```python
from build123d import *

# Parameters (mm, degrees)
BOSS_EXTRUDE1_DEPTH = 22
SKETCH2_R           = 3
BOSS_EXTRUDE2_DEPTH = 14
SKETCH5_R           = 3.63
BOSS_EXTRUDE3_DEPTH = 2
SKETCH7_R           = 1.5
CUT_EXTRUDE1_DEPTH  = 3.5
SKETCH8_R           = 12
BOSS_EXTRUDE4_DEPTH = 31
SKETCH9_R           = 1.5
BOSS_EXTRUDE5_DEPTH = 7
SKETCH10_R          = 4
BOSS_EXTRUDE6_DEPTH = 2
SKETCH11_R          = 1.5
CUT_EXTRUDE2_DEPTH  = 3.5


with BuildPart() as part:
    # Sketch1 → Boss-Extrude1 (new body)
    with BuildSketch(Plane.XY):
        with BuildLine():
            Line((-20.5, -16), (20.5, -16))
            ThreePointArc((20.5, -16), (22.267766953, -15.267766953), (23, -13.5))
            Line((23, -13.5), (23, 13.5))
            ThreePointArc((23, 13.5), (22.267766953, 15.267766953), (20.5, 16))
            Line((20.5, 16), (-20.5, 16))
            ThreePointArc((-20.5, 16), (-22.267766953, 15.267766953), (-23, 13.5))
            Line((-23, 13.5), (-23, -13.5))
            ThreePointArc((-23, -13.5), (-22.267766953, -15.267766953), (-20.5, -16))
        make_face()
    extrude(amount=BOSS_EXTRUDE1_DEPTH)

    # Sketch2 → Boss-Extrude2 (add)
    with BuildSketch(Plane.XY.offset(22)):
        with Locations((-8.2, 0)):
            Circle(SKETCH2_R)
    extrude(amount=BOSS_EXTRUDE2_DEPTH)

    # Sketch5 → Boss-Extrude3 (add)
    with BuildSketch(Plane.XY.offset(22)):
        with Locations((-17.2, 9.11)):
            Circle(SKETCH5_R)
        with Locations((-17.2, -9.09)):
            Circle(SKETCH5_R)
        with Locations((15.8, 9.11)):
            Circle(SKETCH5_R)
        with Locations((15.8, -9.09)):
            Circle(SKETCH5_R)
    extrude(amount=BOSS_EXTRUDE3_DEPTH)

    # Sketch7 → Cut-Extrude1 (cut)
    with BuildSketch(Plane.XY.offset(24)):
        with Locations((-17.2, 9.11)):
            Circle(SKETCH7_R)
        with Locations((-17.2, -9.09)):
            Circle(SKETCH7_R)
        with Locations((15.7, 9.11)):
            Circle(SKETCH7_R)
        with Locations((15.7, -9.09)):
            Circle(SKETCH7_R)
    extrude(amount=-CUT_EXTRUDE1_DEPTH, mode=Mode.SUBTRACT)

    # Sketch8 → Boss-Extrude4 (add)
    with BuildSketch(Plane(origin=(23, 0, 0), x_dir=(0, 0, -1), z_dir=(1, 0, 0))):
        with Locations(Location((-10, 0, 0), (0, 0, 180))):
            Circle(SKETCH8_R)
    extrude(amount=BOSS_EXTRUDE4_DEPTH)

    # Sketch9 → Boss-Extrude5 (add)
    with BuildSketch(Plane(origin=(54, 0, 0), x_dir=(0, 0, -1), z_dir=(1, 0, 0))):
        with Locations((-10, 0)):
            Circle(SKETCH9_R)
    extrude(amount=BOSS_EXTRUDE5_DEPTH)

    # Sketch10 → Boss-Extrude6 (add)
    with BuildSketch(Plane(origin=(57, 0, 0), x_dir=(0, 0, -1), z_dir=(1, 0, 0))):
        with Locations((-10, 0)):
            Circle(SKETCH10_R)
    extrude(amount=BOSS_EXTRUDE6_DEPTH)

    # Sketch11 → Cut-Extrude2 (cut)
    with BuildSketch(Plane.XY.offset(36)):
        with Locations((-8.2, 0)):
            Circle(SKETCH11_R)
    extrude(amount=-CUT_EXTRUDE2_DEPTH, mode=Mode.SUBTRACT)


solid = part.part
```
Geometry check sheet. Reference: the model listing, model coordinates, mm. A direction names the side the tool comes from. Round coordinates to 2 decimals unless told otherwise and drop trailing zeros. Loops run counter-clockwise (first coordinate to the right, second up) from the corner with the lowest first, then second, coordinate; pieces in that order, holes last. Notation, with made-up numbers: (-21, 10.25) -> (36, 10.25) arc R18 cw to (36, 45.25) -> close; hole circle Ø6 at (40, 60.5). An arc over 180 degrees is marked (long way). Use a Markdown table: item, result.
(1) Set-up check for faces 1 (the flat face through (57, -2, 10)), 2 (the cylindrical face through (38.28, -0.53, -1.99)), 3 (the cylindrical face through (-22.287, -15.248, 10.846)), 4 (the cylindrical face through (-15.52, -12.31, 22.99)), 5 (the flat face through (0, -16, 11)): record each of +Z, -Z, +X, -X, +Y, -Y from which the full face is reachable in a straight line by a thin tool's end or side.
Calculated:
| item | result |
|---|---|
| face 1 | none |
| face 2 | +X |
| face 3 | +Z, -Z, -X, -Y |
| face 4 | +Z |
| face 5 | +Z, -Z, +X, -X, -Y |
(2) Go/stop test with flat-tipped pins: P1, Ø3.5, axis at x = -17.5, y = -9, coming from the +Z side; P2, Ø10, axis at x = 15, y = 5.5, coming from the -Z side; P3, Ø6, axis at x = 49, z = 20, coming from the +Y side. Record where each tip stops, or that it passes through.
Calculated:
| item | result |
|---|---|
| P1 | z = 24 |
| P2 | z = 0 |
| P3 | y = 9.75 |
(3) Sectioned sample at A-A (x = -17.2). Enter the section's corners in (y, z), then the cut area to 3 significant figures.
Calculated:
| item | result |
|---|---|
| outline | (-16, 0) -> (16, 0) -> (16, 22) -> (12.74, 22) -> (12.74, 24) -> (10.61, 24) -> (10.61, 20.5) -> (7.61, 20.5) -> (7.61, 24) -> (5.48, 24) -> (5.48, 22) -> (-5.46, 22) -> (-5.46, 24) -> (-7.59, 24) -> (-7.59, 20.5) -> (-10.59, 20.5) -> (-10.59, 24) -> (-12.72, 24) -> (-12.72, 22) -> (-16, 22) -> close |
| area | 712 mm² |
(4) Mould release check, pull along Y, two halves, no side actions. Record for faces 6 (the flat face through (54, 2, 10)), 7 (the flat face through (16, -9, 20.5)), 8 (the cylindrical face through (22.248, -15.287, 10.846)): released by +Y, released by -Y, zero draft, split by the parting line, or undercut.
Calculated:
| item | result |
|---|---|
| face 6 | zero draft |
| face 7 | undercut |
| face 8 | released by -Y |
(5) Sectioned sample at B-B (y = -9.09). Enter the section's corners in (x, z).
Calculated:
| item | result |
|---|---|
| outline | (-23, 0) -> (23, 0) -> (23, 2.17) -> (54, 2.17) -> (54, 17.83) -> (23, 17.83) -> (23, 22) -> (19.43, 22) -> (19.43, 24) -> (17.2, 24) -> (17.2, 20.5) -> (14.2, 20.5) -> (14.2, 24) -> (12.17, 24) -> (12.17, 22) -> (-13.57, 22) -> (-13.57, 24) -> (-15.7, 24) -> (-15.7, 20.5) -> (-18.7, 20.5) -> (-18.7, 24) -> (-20.83, 24) -> (-20.83, 22) -> (-23, 22) -> close |
(6) Scan lines: probe 1 along X at (y, z) = (9, 21); probe 2 along Y at (x, z) = (-17.2, 23); probe 3 along Y at (x, z) = (15.7, 21.4). Record each from-to range of solid material in increasing order.
Calculated:
| item | result |
|---|---|
| probe 1 | -23 to -18.7, -15.7 to 14.2, 17.2 to 23 |
| probe 2 | -12.72 to -10.59, -7.59 to -5.46, 5.48 to 7.61, 10.61 to 12.74 |
| probe 3 | -16 to -10.59, -7.59 to 7.61, 10.61 to 16 |
(7) Sectioned sample at C-C (z = 10). Enter the section's corners in (x, y).
Calculated:
| item | result |
|---|---|
| outline | (-23, -13.5) arc R2.5 ccw to (-20.5, -16) -> (20.5, -16) arc R2.5 ccw to (23, -13.5) -> (23, -12) -> (54, -12) -> (54, -1.5) -> (57, -1.5) -> (57, -4) -> (59, -4) -> (59, -1.5) -> (61, -1.5) -> (61, 1.5) -> (59, 1.5) -> (59, 4) -> (57, 4) -> (57, 1.5) -> (54, 1.5) -> (54, 12) -> (23, 12) -> (23, 13.5) arc R2.5 ccw to (20.5, 16) -> (-20.5, 16) arc R2.5 ccw to (-23, 13.5) -> close |
